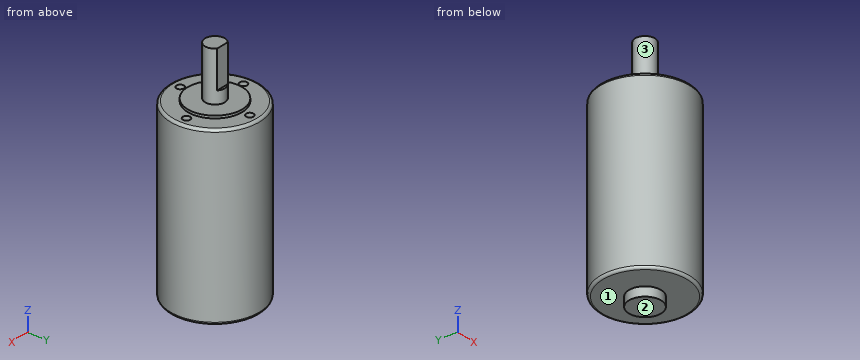
from build123d import *

# Parameters (mm, degrees)
SKETCH1_R           = 18
SKETCH1_R_2         = 1.5
GEAR_DEPTH          = 20
SKETCH2_R           = 18
MOTOR_DEPTH         = 50
SKETCH3_R           = 6.5
BOSS_EXTRUDE3_DEPTH = 3.7
SKETCH4_R           = 11
BOSS_EXTRUDE4_DEPTH = 1
SKETCH5_R           = 4
SHAFT_DEPTH         = 20
CUT_EXTRUDE1_DEPTH  = 15
FILLET1_R           = 1


with BuildPart() as part:
    # Sketch1 → Gear (new body)
    with BuildSketch(Plane.XY):
        Circle(SKETCH1_R)
        with Locations((0, 14)):
            Circle(SKETCH1_R_2, mode=Mode.SUBTRACT)
        with Locations((14, 0)):
            Circle(SKETCH1_R_2, mode=Mode.SUBTRACT)
        with Locations((0, -14)):
            Circle(SKETCH1_R_2, mode=Mode.SUBTRACT)
        with Locations((-14, 0)):
            Circle(SKETCH1_R_2, mode=Mode.SUBTRACT)
    extrude(amount=-GEAR_DEPTH)

    # Sketch2 → Motor (add)
    with BuildSketch(Plane(origin=(0, 0, -20), x_dir=(-1, 0, 0), z_dir=(0, 0, -1))):
        with Locations(Location((0, 0, 0), (0, 0, 180))):
            Circle(SKETCH2_R)
    extrude(amount=MOTOR_DEPTH)

    # Sketch3 → Boss-Extrude3 (add)
    with BuildSketch(Plane(origin=(0, 0, -70), x_dir=(-1, 0, 0), z_dir=(0, 0, -1))):
        Circle(SKETCH3_R)
    extrude(amount=BOSS_EXTRUDE3_DEPTH)

    # Sketch4 → Boss-Extrude4 (add)
    with BuildSketch(Plane.XY):
        Circle(SKETCH4_R)
    extrude(amount=BOSS_EXTRUDE4_DEPTH)

    # Sketch5 → shaft (add)
    with BuildSketch(Plane.XY.offset(1)):
        Circle(SKETCH5_R)
    extrude(amount=SHAFT_DEPTH)

    # Sketch6 → Cut-Extrude1 (cut)
    with BuildSketch(Plane.XY.offset(21)):
        Polygon((-71.543868334, 3), (-2.645751311, 3), (2.645751311, 3), (71.543868334, 3), (71.543868334, 140.796234045), (-71.543868334, 140.796234045), align=None)
    extrude(amount=-CUT_EXTRUDE1_DEPTH, mode=Mode.SUBTRACT)

    # Fillet1
    fillet1_edges = [part.edges().sort_by_distance(p)[0] for p in [
        (-18, 0, 0),
        (-18, 0, -70),
    ]]
    fillet(fillet1_edges, radius=FILLET1_R)


solid = part.part
Geometry check sheet. Reference: the model listing, model coordinates, mm. Face numbers are marked on the shaded views. A direction names the side the tool comes from. Round coordinates to 2 decimals unless told otherwise and drop trailing zeros. Loops run counter-clockwise (first coordinate to the right, second up) from the corner with the lowest first, then second, coordinate; pieces in that order, holes last. Notation, with made-up numbers: (4.5, 49) - (62.5, 49) arc R13 cw to (62.5, 71) - close; hole circle Ø1 at (10.25, 26.25). An arc over 180 degrees is marked (long way). Answer as CSV lines item,"result".
(1) Cross-section at C-C, the plane z = -19. Enter the section's corners in (x, y).
Output values:
outline,"circle Ø36 at (0, 0); hole circle Ø3 at (-14, 0); hole circle Ø3 at (0, -14); hole circle Ø3 at (0, 14); hole circle Ø3 at (14, 0)"
(2) Set-up check for the marked faces 1, 2 and 3: record each of +Z, -Z, +X, -X, +Y, -Y from which the full face is reachable in a straight line by a thin tool's end or side.
Output values:
face 1,"-Z"
face 2,"-Z, +X, -X, +Y, -Y"
face 3,"+Z"
(3) Material ranges on line 1 along X through (y, z) = (0.5, -10); line 2 along Z through (x, y) = (-6, 6); line 3 along Z through (x, y) = (-11.5, -12), recorded low to high.
Output values:
line 1,"x = -17.99 to -15.41, -12.59 to 12.59, 15.41 to 17.99"
line 2,"z = -70 to 1"
line 3,"z = -70 to 0"
(4) Depth check by flat-ended pin: pin 1 Ø1.1 at (x, y) = (0, 3.5) entering from +Z; pin 2 Ø8 at (y, z) = (6.5, -38) entering from -X; pin 3 Ø2 at (x, z) = (-11, -40) entering from -Y; pin 4 Ø2.5 at (x, y) = (0, 14) entering from +Z. Enter the tip coordinate at first touch or a pass-through.
Output values:
pin 1,"stops at z = 21"
pin 2,"stops at x = -17.83"
pin 3,"stops at y = -14.97"
pin 4,"stops at z = -20"
(5) Cross-section at D-D, the plane z = -39.5. Enter the section's corners in (x, y).
Output values:
outline,"circle Ø36 at (0, 0)"
(6) Cross-section at A-A, the plane y = 0. Enter the section's corners in (x, z).
Output values:
outline,"(-18, -69) arc R1 ccw to (-17, -70) - (-6.5, -70) - (-6.5, -73.7) - (6.5, -73.7) - (6.5, -70) - (17, -70) arc R1 ccw to (18, -69) - (18, -1) arc R1 ccw to (17, 0) - (15.5, 0) - (15.5, -20) - (12.5, -20) - (12.5, 0) - (11, 0) - (11, 1) - (4, 1) - (4, 21) - (-4, 21) - (-4, 1) - (-11, 1) - (-11, 0) - (-12.5, 0) - (-12.5, -20) - (-15.5, -20) - (-15.5, 0) - (-17, 0) arc R1 ccw to (-18, -1) - close"
